Source: three-view drawing plus pictorial views. Frame: mm from the lowest corner of the part. A direction names the side the tool comes from. Round coordinates to 2 decimals unless told otherwise and drop trailing zeros. Loops run counter-clockwise (first coordinate to the right, second up) from the corner with the lowest first, then second, coordinate; pieces in that order, holes last. Notation, with made-up numbers: M -9,32.5 L -5,32.5 A22 ccw -5,42.5 Z; hole C -16,-20 d1. An arc over 180 degrees is marked long. Answer as a JSON object with one key per item and string values.
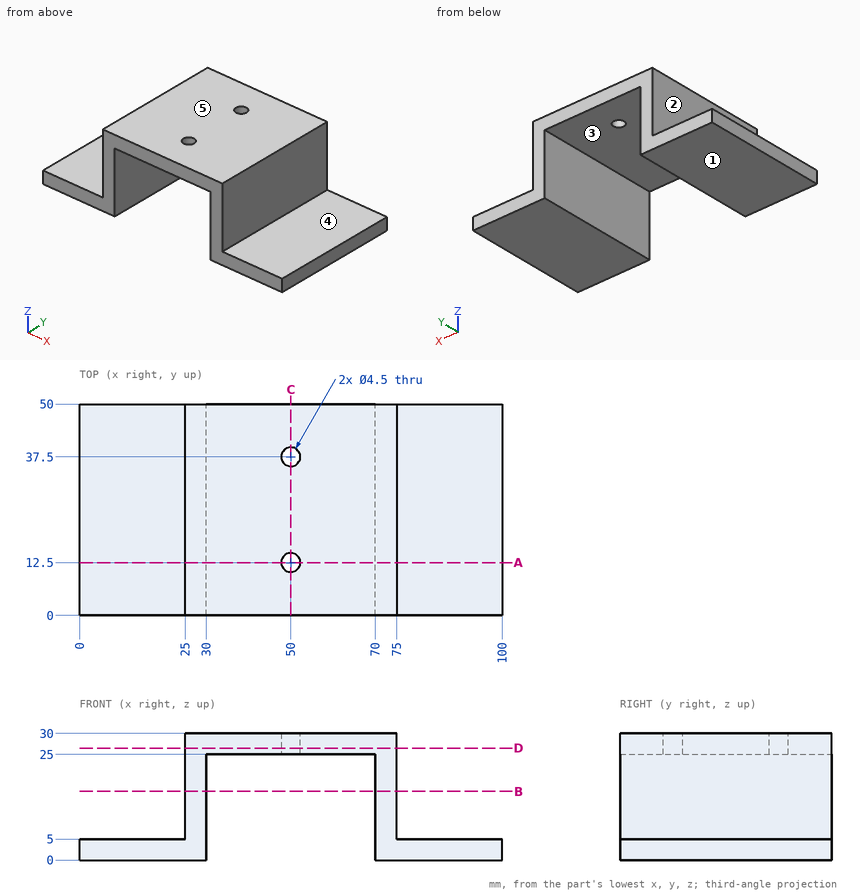
1) Cut plane D-D on z = 26.5. Return the cut outline in (x, y).
Geometry results:
{"outline": "M 25,0 L 75,0 L 75,50 L 25,50 Z; hole C 50,12.5 d4.5; hole C 50,37.5 d4.5"}
2) Cut plane B-B on z = 16.25. Return the cut outline in (x, y), and give its area (3 significant figures).
Geometry results:
{"outline": "M 25,0 L 30,0 L 30,50 L 25,50 Z; M 70,0 L 75,0 L 75,50 L 70,50 Z", "area": "500 mm2"}
3) First-contact query: pin 1 (8 mm diameter, centred on y = 11, z = 23.5, fed in from -X); pin 2 (20 mm diameter, centred on x = 88.5, y = 36, fed in from +Z); pin 3 (12 mm diameter, centred on x = 51.5, y = 21.5, fed in from -Z). Flat tips, straight axial feed; report the tip coordinate or a pass-through.
Geometry results:
{"pin 1": "x = 25", "pin 2": "z = 5", "pin 3": "z = 25"}
4) Line query: probe 1 along Y at (x, z) = (50, 28.8); probe 2 along X at (y, z) = (23.5, 5.5); probe 3 along X at (y, z) = (32, 2.5). Output: solid intervals per line, ascending.
Geometry results:
{"probe 1": "0 to 10.25, 14.75 to 35.25, 39.75 to 50", "probe 2": "25 to 30, 70 to 75", "probe 3": "0 to 30, 70 to 100"}
5) Set-up query: the marked faces 1, 2, 3, 4 and 5. Return all of +Z, -Z, +X, -X, +Y, -Y with unobstructed straight access to the full face (end or side cutting, diameter ignored); none if empty.
Geometry results:
{"face 1": "-Z, +X, -X, +Y, -Y", "face 2": "+Z, -X, +Y, -Y", "face 3": "-Z, +Y, -Y", "face 4": "+Z, +X, +Y, -Y", "face 5": "+Z, +X, -X, +Y, -Y"}
6) Cut plane C-C on x = 50. Return the cut outline in (y, z), and give its area (3 significant figures).
Geometry results:
{"outline": "M 0,25 L 10.25,25 L 10.25,30 L 0,30 Z; M 14.75,25 L 35.25,25 L 35.25,30 L 14.75,30 Z; M 39.75,25 L 50,25 L 50,30 L 39.75,30 Z", "area": "205 mm2"}
7) Cut plane A-A on y = 12.5. Return the cut outline in (x, z), and give its area (4 significant figures).
Geometry results:
{"outline": "M 0,0 L 30,0 L 30,25 L 47.75,25 L 47.75,30 L 25,30 L 25,5 L 0,5 Z; M 52.25,25 L 70,25 L 70,0 L 100,0 L 100,5 L 75,5 L 75,30 L 52.25,30 Z", "area": "727.5 mm2"}
